The model under review builds one solid part; all positions refer to its coordinate system, in mm. Face numbers are marked on the shaded views. Round coordinates to 2 decimals unless told otherwise and drop trailing zeros. Order: outer loops, then holes, each group sorted by start corner. A loop starts at its lowest first (then second) coordinate and runs counter-clockwise, first axis right, second up. Notation, with made-up numbers: M 16.25,64 L 65.25,64 A17 cw 65.25,78 Z; hole C -7,-39 d3. An arc over 180 degrees is marked long. Answer as a JSON object with one key per item and string values. Group by question number.
1. Add section B-B on z = -0.95. State the section outline as (x, y) points.
2. Clearance check with flat-ended pins moving along their axes: P1, Ø1.5, axis at y = 43.5, z = -2, coming from the +X side; P2, Ø2, axis at x = 1, z = 0, coming from the +Y side; P3, Ø1.5, axis at x = 1.5, y = 36, coming from the -Z side. State where each tip first meets the part, or that it passes through.
3. Add section A-A on x = 0. State the section outline as (y, z) points.
4. Mouldability with a two-part tool opening along X and no side actions: class the marked faces 1, 2 and 3 as released by +X, released by -X, zero draft, split by the parting line, or undercut.
5. To check wall thickness, follow probe 1 along Y at (x, z) = (-2.6, -0.5); probe 2 along X at (y, z) = (18, 0.15). State the ranges of each line that lie inside material, in increasing order. Write a range as [from, to].
6. Add section C-C on y = 27. State the section outline as (x, z) points, and give its area (3 significant figures).
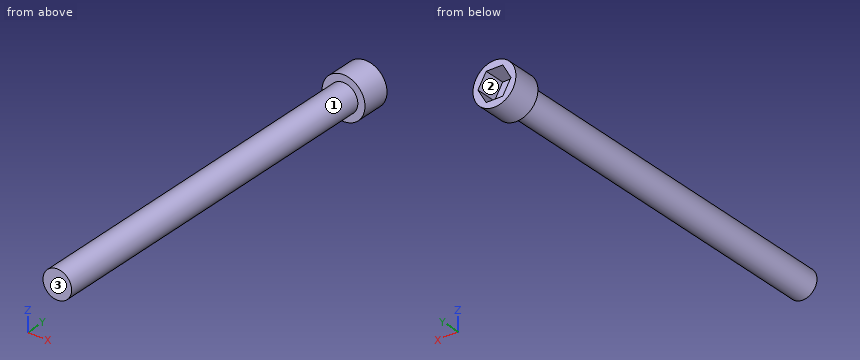
Autodesk Inventor part; units mm, degrees
ref_plane "YZ Plane" through (0, 0, 0) normal (1, 0, 0) x (0, 1, 0)
ref_plane "XZ Plane" through (0, 0, 0) normal (0, 1, 0) x (-1, 0, 0)
ref_plane "XY Plane" through (0, 0, 0) normal (0, 0, 1) x (1, 0, 0)
sketch "Sketch1" plane through (0, 0, 0) normal (0, 1, 0) x (-1, 0, 0)
  circle A0 centre (0, 0) radius 2
  dimension "d0" = 4
extrude "Extrusion1" add sketch "Sketch1" along normal blind 52
thread "Thread1"
sketch "Sketch2" plane through (0, 52, 0) normal (0, 1, 0) x (1, 0, 0)
  circle A0 centre (0, 0) radius 3
  dimension "d5" = 6
extrude "Extrusion2" add sketch "Sketch2" along normal blind 4
sketch "Sketch3" plane through (0, 56, 0) normal (0, 1, 0) x (1, 0, 0)
  circle A0 centre (0, 0) radius 2
  line L0 (1.1547, 2) -> (2.3094, 0)
  line L1 (2.3094, 0) -> (1.1547, -2)
  line L2 (1.1547, -2) -> (-1.1547, -2)
  line L3 (-1.1547, -2) -> (-2.3094, 0)
  line L4 (-2.3094, 0) -> (-1.1547, 2)
  line L5 (-1.1547, 2) -> (1.1547, 2)
  point P0 (0, 2)
extrude "Extrusion3" cut sketch "Sketch3" against normal blind 3
properties part number "New Bolt" material "Steel"
Recorded:
{
 "1": {"outline": "M -2.85,52 L -1.76,52 L -1.76,0 L 1.76,0 L 1.76,52 L 2.85,52 L 2.85,56 L 1.76,56 L 1.76,53 L -1.76,53 L -1.76,56 L -2.85,56 Z"},
 "2": {"P1": "stops at x = 1.56", "P2": "stops at y = 53", "P3": "stops at z = -1.85"},
 "3": {"outline": "M 0,-2 L 52,-2 L 52,-3 L 56,-3 L 56,-2 L 53,-2 L 53,2 L 56,2 L 56,3 L 52,3 L 52,2 L 0,2 Z"},
 "4": {"face 1": "split by the parting line", "face 2": "undercut", "face 3": "zero draft"},
 "5": {"probe 1": "y = [52, 56]", "probe 2": "x = [-1.99, 1.99]"},
 "6": {"outline": "C 0,0 d4", "area": "12.6 mm²"}
}
